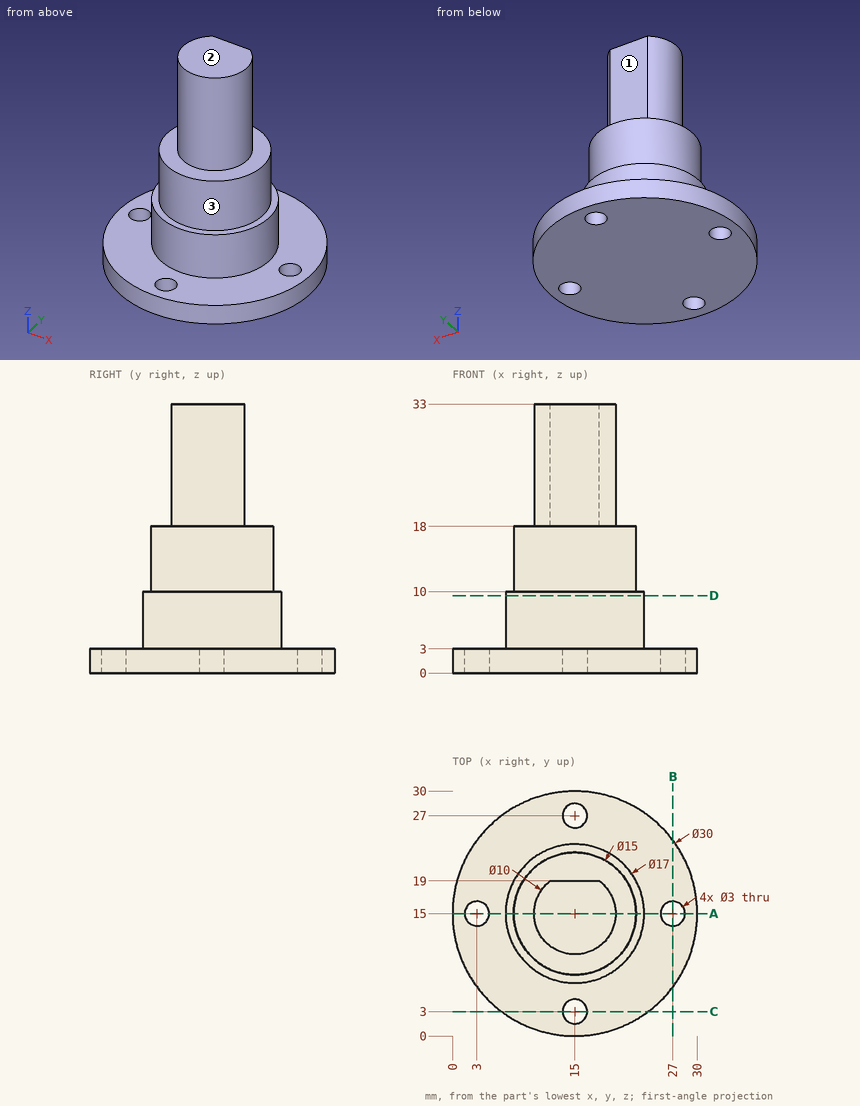
For this review, use the dimensioned drawing (mm, ordinates from the lowest corner) and the shaded views. A direction names the side the tool comes from. Round coordinates to 2 decimals unless told otherwise and drop trailing zeros. Order: outer loops, then holes, each group sorted by start corner. A loop starts at its lowest first (then second) coordinate and runs counter-clockwise, first axis right, second up. Notation, with made-up numbers: (-39.75, 79.25) -> (-28.75, 79.25) arc R27 ccw to (-28.75, 116.25) -> close; hole circle Ø1 at (33.5, 34). An arc over 180 degrees is marked (long way). Use CSV: the item, a comma, the result in double quotes. Start each with the question number.
(1) Tool access review of the marked faces 1, 2 and 3: name each direction out of +Z, -Z, +X, -X, +Y, -Y from which nothing blocks a thin tool from reaching the whole face with its end or side.
(2) Consider section D-D on z = 9.5. Write out the cut boundary in (x, y).
(3) Consider section B-B on x = 27. Write out the cut boundary in (y, z), and give its area (3 significant figures).
(4) Consider section A-A on y = 15. Write out the cut boundary in (x, z), and give its area (3 significant figures).
(5) Wall thickness on probe 1 along Z at (x, y) = (15.25, 25.25); probe 2 along Z at (x, y) = (10.25, 18.5); probe 3 along X at (y, z) = (15, 15.5): over which ranges is each line inside the solid? List them lowest first. Write a range as from..to.
(6) Insertion check: pin 1 (2 mm diameter, centred on x = 7, y = 14.5, fed in from +Z); pin 2 (1.5 mm diameter, centred on x = 17.5, z = 7.5, fed in from +Y); pin 3 (1.8 mm diameter, centred on x = 15.5, z = 27, fed in from +Y). Each pin has a flat end and moves straight along its axis. Give the tip position at first contact, or say it passes through.
Responses:
1,face 1,"+Z, +X, -X, +Y"
1,face 2,"+Z, +X, -X, +Y, -Y"
1,face 3,"+Z"
2,outline,"circle Ø17 at (15, 15)"
3,outline,"(6, 0) -> (13.5, 0) -> (13.5, 3) -> (6, 3) -> close; (16.5, 0) -> (24, 0) -> (24, 3) -> (16.5, 3) -> close"
3,area,"45.0 mm²"
4,outline,"(0, 0) -> (1.5, 0) -> (1.5, 3) -> (0, 3) -> close; (4.5, 0) -> (25.5, 0) -> (25.5, 3) -> (23.5, 3) -> (23.5, 10) -> (22.5, 10) -> (22.5, 18) -> (20, 18) -> (20, 33) -> (10, 33) -> (10, 18) -> (7.5, 18) -> (7.5, 10) -> (6.5, 10) -> (6.5, 3) -> (4.5, 3) -> close; (28.5, 0) -> (30, 0) -> (30, 3) -> (28.5, 3) -> close"
4,area,"461 mm²"
5,probe 1,"0..3"
5,probe 2,"0..18"
5,probe 3,"7.5..22.5"
6,pin 1,"z = 18"
6,pin 2,"y = 23.32"
6,pin 3,"y = 19"
